Model file for the job. Use its own axes, mm. A direction names the side the tool comes from. Give positions to 0.01 mm unless a question says otherwise; leave off trailing zeros. Write each loop counter-clockwise with the first axis right and the second up, starting at its lowest first coordinate (ties: lowest second). Pieces come first, ordered by that corner, then holes. Notation, with made-up numbers: M 74.25,-4 L 128.25,-4 A25 cw 128.25,24 Z; hole C 88.5,-27.5 d9. An arc over 180 degrees is marked long. Answer as a JSON object with one key per item and string values. Group by question number.
```python
from build123d import *

# Parameters (mm, degrees)
ESQUISSE2_R             = 2
ENL_V_MAT_EXTRU_1_DEPTH = 5


with BuildPart() as part:
    # Esquisse1 → Révolution1 (revolve)
    with BuildSketch(Plane.XY):
        with BuildLine():
            Line((16.6, 16.5), (3.15, 16.5))
            Line((3.15, 16.5), (3.15, 0))
            Line((3.15, 0), (5.55, 0))
            Line((5.55, 0), (5.55, 10))
            ThreePointArc((5.55, 10), (6.282233047, 11.767766953), (8.05, 12.5))
            Line((8.05, 12.5), (16.6, 12.5))
            Line((16.6, 12.5), (16.6, 16.5))
        make_face()
    revolve(axis=Axis((0, 0, 0), (0, 1, 0)))

    # Esquisse2 → Enlèv. mat.-Extru.1 (cut, through all)
    with BuildSketch(Plane.XZ.offset(-12.5)):
        with Locations((0, 11.75)):
            Circle(ESQUISSE2_R)
        with Locations((10.175798494, -5.875)):
            Circle(ESQUISSE2_R)
        with Locations((-10.175798494, -5.875)):
            Circle(ESQUISSE2_R)
    extrude(amount=-ENL_V_MAT_EXTRU_1_DEPTH, mode=Mode.SUBTRACT)


solid = part.part
```
Q1. 3-axis set-ups, long thin cutter, end or side, ignore diameter. For faces 1 (the cylindrical face through (2.98, 5.07, -4.68)), 2 (the cylindrical face through (-3.599, 14.528, 16.205)): which of +Z, -Z, +X, -X, +Y, -Y reach the whole face in a straight line?
Q2. Drop flat-ended pins along their axis: P1, Ø5, axis at x = -6.5, y = 12.5, coming from the -Z side; P2, Ø5, axis at x = 5.5, y = 5, coming from the -Z side; P3, Ø3, axis at y = 12.5, z = -8, coming from the +X side. Give the stop position or say it passes through.
Q3. Slice it at C-C, the plane y = 4. Write the cut outline in (x, z), then the cut area to 3 significant figures.
Q4. Slice it at D-D, the plane y = 13. Write the cut outline in (x, z) (3 decimals), then the cut area to 3 significant figures.
Q5. Wall check: L1, parallel to X at y = 4.5, z = 0; L2, parallel to Y at x = -14.5, z = 0; L3, parallel to Z at x = 1.5, y = 12.75. Give the ranges that are in metal, low to high.
Q6. Slice it at A-A, the plane x = 0. Write the cut outline in (y, z).
Q7. Slice it at B-B, the plane z = 0. Write the cut outline in (x, y).
Solved:
{
 "1": {"face 1": "-Y", "face 2": "+Y, -Y"},
 "2": {"P1": "stops at z = -16.11", "P2": "stops at z = -4.67", "P3": "stops at x = 15.27"},
 "3": {"outline": "C 0,0 d11.1; hole C 0,0 d6.3", "area": "65.6 mm²"},
 "4": {"outline": "C 0,0 d33.2; hole C -10.176,-5.875 d4; hole C 0,0 d6.3; hole C 0,11.75 d4; hole C 10.176,-5.875 d4", "area": "797 mm²"},
 "5": {"L1": "x = -5.55 to -3.15, 3.15 to 5.55", "L2": "y = 12.5 to 16.5", "L3": "z = -16.53 to -2.77, 2.77 to 10.43, 13.07 to 16.53"},
 "6": {"outline": "M 0,-5.55 L 10,-5.55 A2.5 cw 12.5,-8.05 L 12.5,-16.6 L 16.5,-16.6 L 16.5,-3.15 L 0,-3.15 Z; M 0,3.15 L 16.5,3.15 L 16.5,9.75 L 12.5,9.75 L 12.5,8.05 A2.5 cw 10,5.55 L 0,5.55 Z; M 12.5,13.75 L 16.5,13.75 L 16.5,16.6 L 12.5,16.6 Z"},
 "7": {"outline": "M -16.6,12.5 L -8.05,12.5 A2.5 cw -5.55,10 L -5.55,0 L -3.15,0 L -3.15,16.5 L -16.6,16.5 Z; M 3.15,0 L 5.55,0 L 5.55,10 A2.5 cw 8.05,12.5 L 16.6,12.5 L 16.6,16.5 L 3.15,16.5 Z"}
}
